Here's how the part is built. I have some questions about the finished solid (model axes, mm). A direction names the side the tool comes from. Round coordinates to 2 decimals unless told otherwise and drop trailing zeros. Write each loop counter-clockwise with the first axis right and the second up, starting at its lowest first coordinate (ties: lowest second). Pieces come first, ordered by that corner, then holes. Notation, with made-up numbers: (32.25, 8.25) -> (69.25, 8.25) arc R25 cw to (69.25, 24.25) -> close; hole circle Ø4 at (-11, 58). An arc over 180 degrees is marked (long way). Put each result on its own line as item: value. Start each with the question number.
1. Suppose I cut it at D-D (x = 353). Please give me the cut outline in (y, z).
2. I need wall thicknesses on probe 1 along X at (y, z) = (10.5, 122.5); probe 2 along Y at (x, z) = (371, 5); probe 3 along Z at (x, y) = (250, -1.75). Which ranges of each line are inside material? Lowest first, please. Write a range as from..to.
3. For pin 1 (2 mm diameter, centred on y = 7, z = -24.5, fed in from -X); pin 2 (2 mm diameter, centred on y = 8, z = -34.5, fed in from -X); pin 3 (23.5 mm diameter, centred on x = 289.5, z = 82.5, fed in from -Y), each with a flat end and sliding along its axis, tell me the tip position at first contact or that it passes through.
4. Suppose I cut it at C-C (z = 83). Please give me the cut outline in (x, y).
5. Suppose I cut it at B-B (x = 404.5). Please give me the cut outline in (y, z), then the cut area to 3 significant figures.
6. Suppose I cut it at A-A (y = 5). Please give me the cut outline in (x, z).
7. Which directions (+Z, -Z, +X, -X, +Y, -Y) give clear straight access to the entire face, cutting with the end or side of a thin tool? Please do faces 4 (the face through (249.14, -1.52, 126.59)), 5 (the face through (447, 11, 127)), 6 (the face through (347, 6, -43.666)), 7 (the face through (341.765, 3.902, -54.054)), 8 (the face through (279.925, 0.168, 59.728)).
8. We'd pull the mould along Z, two halves only. Please class faces 1 (the face through (366, -3, -33)), 2 (the face through (357, 0, -9)), 3 (the face through (287.747, 3.902, 33.508)): +Z half, -Z half, draft (parallel to the pull), parting line (faces both ways), or undercut.
```python
from build123d import *

# Parameters (mm, degrees)
BOSS_EXTRUDE1_DEPTH      = 1
BOSS_EXTRUDE2_DEPTH      = 11
BOSS_EXTRUDE3_DEPTH      = 5
BOSS_EXTRUDE3_DEPTH_BACK = 3
SKETCH3_W                = 50
SKETCH3_H                = 7
CUT_EXTRUDE3_DEPTH       = 25
SKETCH5_W                = 50
SKETCH5_H                = 7
CUT_EXTRUDE4_DEPTH       = 25
SKETCH6_W                = 50
SKETCH6_H                = 7
CUT_EXTRUDE5_DEPTH       = 25


with BuildPart() as part:
    # Sketch1 → Boss-Extrude1 (new body)
    with BuildSketch(Plane(origin=(0, 0, 0), x_dir=(1, 0, 0), z_dir=(0, 1, 0))):
        Polygon((243.304219773, -116.484791866), (254.809280576, -136.408896139), (442.602090749, -136.409305398), (444.621046679, -132.925433223), (441.749040748, -132.925433223), (449.516726723, -119.471406457), (450.964695297, -121.978953122), (452.699916621, -118.984688017), (358.778179035, 43.666038066), (335.767496284, 43.666038066), align=None)
        Polygon((428.113670919, -116.417164681), (266.439108268, -116.428009241), (347.273609729, 23.609230825), align=None, mode=Mode.SUBTRACT)
    extrude(amount=BOSS_EXTRUDE1_DEPTH)

    # Sketch1<9> → Boss-Extrude2 (add)
    # profile 1 of 2: a face of its own
    with BuildSketch(Plane(origin=(0, 0, 0), x_dir=(1, 0, 0), z_dir=(0, 1, 0))):
        Polygon((229.159432547, -134.984249184), (231.716666588, -139.412373829), (462.829865412, -139.412373829), (465.38624875, -134.984588004), (349.829542096, 65.165499075), (344.716133219, 65.165499075), align=None)
        Polygon((251.922647988, -136.4093054), (233.446303399, -136.408896139), (232.623553959, -134.984217358), (241.860901688, -118.984688019), align=None, mode=Mode.SUBTRACT)
        Polygon((442.602090749, -136.409305398), (254.809280576, -136.408896139), (243.304219773, -116.484791866), (335.767496284, 43.666038066), (358.778179035, 43.666038066), (461.938967957, -134.984588004), (461.116393748, -136.409305398), align=None, mode=Mode.SUBTRACT)
        Polygon((348.096628302, 62.164013367), (357.334800991, 46.166038067), (337.210874326, 46.166038067), (346.44844193, 62.165948237), align=None, mode=Mode.SUBTRACT)
    # profile 2 of 2: a face of its own
    with BuildSketch(Plane(origin=(0, 0, 0), x_dir=(1, 0, 0), z_dir=(0, 1, 0))):
        Polygon((441.749040748, -132.925433223), (444.621046679, -132.925433223), (450.964695297, -121.978953122), (449.516726723, -119.471406457), align=None)
    extrude(amount=BOSS_EXTRUDE2_DEPTH)

    # Sketch1<10> → Boss-Extrude3 (add, two sides: drawn at the far end of the back side and taken through both)
    with BuildSketch(Plane(origin=(0, 0, 0), x_dir=(1, 0, 0), z_dir=(0, 1, 0)).offset(-BOSS_EXTRUDE3_DEPTH_BACK)):
        Polygon((229.159432547, -134.984249184), (231.716666588, -139.412373829), (462.829865412, -139.412373829), (465.38624875, -134.984588004), (349.829542096, 65.165499075), (344.716133219, 65.165499075), align=None)
        Polygon((251.922647988, -136.4093054), (233.446303399, -136.408896139), (232.623553959, -134.984217358), (241.860901688, -118.984688019), align=None, mode=Mode.SUBTRACT)
        Polygon((442.602090749, -136.409305398), (254.809280576, -136.408896139), (243.304219773, -116.484791866), (335.767496284, 43.666038066), (358.778179035, 43.666038066), (452.699916621, -118.984688017), (461.938967957, -134.984588004), (461.116393748, -136.409305398), align=None, mode=Mode.SUBTRACT)
        Polygon((348.096628302, 62.164013367), (357.334800991, 46.166038067), (337.210874326, 46.166038067), (346.44844193, 62.165948237), align=None, mode=Mode.SUBTRACT)
    extrude(amount=BOSS_EXTRUDE3_DEPTH + BOSS_EXTRUDE3_DEPTH_BACK)

    # Sketch3 → Cut-Extrude3 (cut)
    with BuildSketch(Plane(origin=(290.589645397, 0, -167.772009994), x_dir=(-0.49999999999998745, 0, -0.8660254037844459), z_dir=(0.8660254037844459, 0, -0.49999999999998745))):
        with Locations((-236.592990632, -3)):
            Rectangle(SKETCH3_W, SKETCH3_H)
    extrude(amount=-CUT_EXTRUDE3_DEPTH, mode=Mode.SUBTRACT)

    # Sketch5 → Cut-Extrude4 (cut)
    with BuildSketch(Plane.XY.offset(139.412373829)):
        with Locations((347.273266, -3)):
            Rectangle(SKETCH5_W, SKETCH5_H)
    extrude(amount=-CUT_EXTRUDE4_DEPTH, mode=Mode.SUBTRACT)

    # Sketch6 → Cut-Extrude5 (cut)
    with BuildSketch(Plane(origin=(230.319375797, 0, 132.975171838), x_dir=(-0.5000006154012504, 0, 0.8660250484820695), z_dir=(-0.8660250484820695, 0, -0.5000006154012504))):
        with Locations((-113.2366748, -3)):
            Rectangle(SKETCH6_W, SKETCH6_H)
    extrude(amount=-CUT_EXTRUDE5_DEPTH, mode=Mode.SUBTRACT)


solid = part.part
```
Verdict:
1. outline: (-3, -59.67) -> (11, -59.67) -> (11, -53.67) -> (-3, -53.67) -> close; (-3, -46.17) -> (11, -46.17) -> (11, -43.67) -> (1, -43.67) -> (1, -13.69) -> (0, -13.69) -> (0, -43.67) -> (-3, -43.67) -> close; (0.5, 116.42) -> (1, 116.42) -> (1, 136.41) -> (11, 136.41) -> (11, 139.41) -> (0.5, 139.41) -> close
2. probe 1: x = 236.37..239.83, 243.89..246.78, 447.77..450.66, 454.73..458.18
2. probe 2: y = 0..1
2. probe 3: z = 98.89..104.89, 128.08..133.08, 136.41..139.41
3. pin 1: stops at x = 320.66
3. pin 2: stops at x = 326.43
3. pin 3: stops at y = 0
4. outline: (259.17, -3) -> (262.64, -3) -> (262.64, 0) -> (285.73, 0) -> (285.73, 1) -> (262.64, 1) -> (262.64, 11) -> (259.17, 11) -> close; (408.82, 0) -> (431.92, 0) -> (431.92, -3) -> (435.37, -3) -> (435.37, 11) -> (431.92, 11) -> (431.92, 1) -> (408.82, 1) -> close
5. outline: (-3, 136.41) -> (0, 136.41) -> (0, 116.42) -> (1, 116.42) -> (1, 136.41) -> (11, 136.41) -> (11, 139.41) -> (-3, 139.41) -> close; (0, 68.52) -> (0.5, 68.52) -> (0.5, 29.53) -> (11, 29.53) -> (11, 35.51) -> (1, 35.51) -> (1, 75.51) -> (0, 75.51) -> close
5. area: 148 mm^2
6. outline: (229.16, 134.98) -> (344.72, -65.17) -> (349.83, -65.17) -> (465.39, 134.98) -> (462.83, 139.41) -> (231.72, 139.41) -> close; (441.75, 132.93) -> (449.52, 119.47) -> (450.96, 121.98) -> (444.62, 132.93) -> close; hole (232.62, 134.98) -> (241.86, 118.98) -> (251.92, 136.41) -> (233.45, 136.41) -> close; hole (243.3, 116.48) -> (335.77, -43.67) -> (358.78, -43.67) -> (461.94, 134.98) -> (461.12, 136.41) -> (442.6, 136.41) -> (254.81, 136.41) -> close; hole (337.21, -46.17) -> (346.45, -62.17) -> (348.1, -62.16) -> (357.33, -46.17) -> close
7. face 4: -Y
7. face 5: +Z, -Z, +X, -X, +Y
7. face 6: +Y
7. face 7: +Y, -Y
7. face 8: -Z, -Y
8. face 1: draft
8. face 2: undercut
8. face 3: -Z half
